Could you check a few things on this model? Use its own coordinates, in mm. A direction names the side the tool comes from. Coordinates: 2 decimals unless noted, no trailing zeros. Write each loop counter-clockwise with the first axis right and the second up, starting at its lowest first coordinate (ties: lowest second). Pieces come first, ordered by that corner, then holes.
Item 1: I want a section at C-C on x = -10. Please give me the cut outline in (y, z), then the cut area to 3 significant figures.
Item 2: I want a section at B-B on y = 0. Please give me the cut outline in (x, z), then the cut area to 3 significant figures.
Item 3: I want a section at A-A on x = 0. Please give me the cut outline in (y, z).
Item 4: Thinking about a two-plate mould opening in X: for faces 6 (the flat face through (-6, 4, 61)), 7 (the cylindrical face through (0.275, -0.056, 72.497)), 8 (the cylindrical face through (3, 0, 64)), which applies, +X half, -X half, draft (parallel to the pull), parting line (faces both ways), or undercut?
Item 5: If I drill on probe 1 along Z at (x, y) = (0, -2.5); probe 2 along Z at (x, y) = (-1.5, 7); probe 3 along Y at (x, z) = (0.5, 24.5), over which ranges is the centre line in solid material (lowest first)?
Item 6: For P1, Ø9, axis at y = -0.5, z = 55, coming from the +X side; P2, Ø8, axis at x = 0, z = 60, coming from the +Y side; P3, Ø2, axis at y = -11.5, z = -16.5, coming from the +X side; P4, Ø7, axis at x = 3.5, z = 57, coming from the -Y side, each with a flat end and sliding along its axis, tell me the tip position at first contact or that it passes through.
Item 7: Which directions (+Z, -Z, +X, -X, +Y, -Y) give clear straight access to the entire face, cutting with the end or side of a thin tool? Please do faces 1 (the flat face through (-6, -4, 61)), 2 (the cylindrical face through (6.691, -12.864, 0.7)), 3 (the flat face through (12.5, 0, 55)), 4 (the flat face through (-12.5, 0, 55)), 5 (the flat face through (0, 0, -50)).
Item 8: I want a section at D-D on z = 53.5. Please give me the cut outline in (x, y).
from build123d import *

# Parameters (mm, degrees)
F0_R     = 14.5
F1_DEPTH = 50
F2_W     = 25
F2_H     = 8
F3_DEPTH = 10
F5_DEPTH = 8
F6_R     = 5
F7_DEPTH = 25


with BuildPart() as f1:
    # F0 (on Top) → F1 (new body, symmetric)
    with BuildSketch(Plane.XY):
        Circle(F0_R)
    extrude(amount=F1_DEPTH, both=True)

    # F2 (on face) → F3 (join)
    with BuildSketch(Plane.XY.offset(50)):
        Rectangle(F2_W, F2_H)
    extrude(amount=F3_DEPTH)

    # F4 (on face) → F5 (join)
    with BuildSketch(Plane.XZ.offset(4)):
        with BuildLine():
            Line((-12.5, 60), (12.5, 60))
            ThreePointArc((12.5, 60), (0, 72.5), (-12.5, 60))
        make_face()
    extrude(amount=-F5_DEPTH)

    # F6 (on face) → F7 (cut)
    with BuildSketch(Plane.XZ.offset(4)):
        with Locations((0, 60)):
            Circle(F6_R)
    extrude(amount=-F7_DEPTH, mode=Mode.SUBTRACT)


solid = f1.part
Response values:
1. outline: (-10.5, -50) - (10.5, -50) - (10.5, 50) - (4, 50) - (4, 67.5) - (-4, 67.5) - (-4, 50) - (-10.5, 50) - close
1. area: 2,240 mm2
2. outline: (-14.5, -50) - (14.5, -50) - (14.5, 50) - (12.5, 50) - (12.5, 60) arc R12.5 ccw to (-12.5, 60) - (-12.5, 50) - (-14.5, 50) - close; hole circle Ø10 at (0, 60)
2. area: 3,320 mm2
3. outline: (-14.5, -50) - (14.5, -50) - (14.5, 50) - (4, 50) - (4, 55) - (-4, 55) - (-4, 50) - (-14.5, 50) - close; (-4, 65) - (4, 65) - (4, 72.5) - (-4, 72.5) - close
4. face 6: draft
4. face 7: parting line
4. face 8: undercut
5. probe 1: z = -50 to 55, 65 to 72.5
5. probe 2: z = -50 to 50
5. probe 3: y = -14.49 to 14.49
6. P1: stops at x = 12.5
6. P2: passes through
6. P3: stops at x = 10
6. P4: stops at y = -4
7. face 1: +Z, +X, -X, -Y
7. face 2: +Z, -Z
7. face 3: +Z, +X, +Y, -Y
7. face 4: +Z, -X, +Y, -Y
7. face 5: -Z, +X, -X, +Y, -Y
8. outline: (-12.5, -4) - (12.5, -4) - (12.5, 4) - (-12.5, 4) - close
